from build123d import *

# Parameters (mm, degrees)
SKETCH1_R               = 2.485
SKETCH1_R_2             = 2.6
BOSS_EXTRUDE1_DEPTH     = 6
SKETCH2_R               = 2.485
BOSS_EXTRUDE2_DEPTH     = 2
SKETCH3_R               = 1.6
CUT_EXTRUDE1_DEPTH      = 10
SKETCH4_R               = 3
CUT_EXTRUDE2_DEPTH      = 28.03
BOSS_EXTRUDE3_DEPTH     = 20.015
SKETCH6_R               = 2.485
CUT_EXTRUDE3_DEPTH      = 10
CUT_EXTRUDE6_DEPTH      = 91.116192357
CUT_EXTRUDE6_DEPTH_BACK = 6
SKETCH10_R              = 1.485
SKETCH9_R               = 3
SKETCH9_R_2             = 1.485
SKETCH9_R_3             = 2.6
SKETCH9_R_4             = 1.6
CUT_EXTRUDE5_DEPTH      = 109.243744046
FILLET1_R               = 1.5


with BuildPart() as part:
    # Sketch1 → Boss-Extrude1 (new, symmetric)
    with BuildSketch(Plane(origin=(0, 0, 0), x_dir=(1, 0, 0), z_dir=(0, 1, 0))):
        with BuildLine():
            Line((20.015, -4.1), (20.015, -10.015))
            Line((20.015, -10.015), (-20.015, -10.015))
            Line((-20.015, -10.015), (-20.015, 10.015))
            Line((-20.015, 10.015), (20.015, 10.015))
            Line((20.015, 10.015), (20.015, 4.1))
            ThreePointArc((20.015, 4.1), (21.182179477, 1.282179477), (24, 0.115))
            Line((24, 0.115), (29.985, 0.115))
            Line((29.985, 0.115), (29.985, 14.015))
            Line((29.985, 14.015), (-29.985, 14.015))
            Line((-29.985, 14.015), (-29.985, 7.6))
            Line((-29.985, 7.6), (-37.485, 7.6))
            ThreePointArc((-37.485, 7.6), (-45.085, 0), (-37.485, -7.6))
            Line((-37.485, -7.6), (-29.985, -7.6))
            Line((-29.985, -7.6), (-29.985, -88.485))
            Line((-29.985, -88.485), (17.515, -88.485))
            Line((17.515, -88.485), (17.515, -78.515))
            Line((17.515, -78.515), (-20.015, -78.515))
            Line((-20.015, -78.515), (-20.015, -18.015))
            Line((-20.015, -18.015), (29.985, -18.015))
            Line((29.985, -18.015), (29.985, -0.115))
            Line((29.985, -0.115), (24, -0.115))
            ThreePointArc((24, -0.115), (21.182179477, -1.282179477), (20.015, -4.1))
        make_face()
        with Locations(Location((-24, -5, 0), (0, 0, 270))):
            Circle(SKETCH1_R, mode=Mode.SUBTRACT)
        with Locations(Location((-24, 5, 0), (0, 0, 270))):
            Circle(SKETCH1_R, mode=Mode.SUBTRACT)
        with Locations(Location((24, -5, 0), (0, 0, 270))):
            Circle(SKETCH1_R, mode=Mode.SUBTRACT)
        with Locations(Location((24, 5, 0), (0, 0, 270))):
            Circle(SKETCH1_R, mode=Mode.SUBTRACT)
        with Locations(Location((-37.485, 0, 0), (0, 0, 270))):
            Circle(SKETCH1_R_2, mode=Mode.SUBTRACT)
    extrude(amount=BOSS_EXTRUDE1_DEPTH, both=True)

    # Sketch2 → Boss-Extrude2 (add)
    with BuildSketch(Plane.XZ.offset(6)):
        with Locations(Location((24, -5, 0), (0, 0, 90))):
            Circle(SKETCH2_R)
        with Locations(Location((24, 5, 0), (0, 0, 90))):
            Circle(SKETCH2_R)
        with Locations(Location((-24, -5, 0), (0, 0, 90))):
            Circle(SKETCH2_R)
        with Locations(Location((-24, 5, 0), (0, 0, 90))):
            Circle(SKETCH2_R)
    extrude(amount=-BOSS_EXTRUDE2_DEPTH)

    # Sketch3 → Cut-Extrude1 (cut)
    with BuildSketch(Plane.XY.offset(18.015)):
        with Locations((10.015, 0)):
            Circle(SKETCH3_R)
    extrude(amount=-CUT_EXTRUDE1_DEPTH, mode=Mode.SUBTRACT)

    # Sketch4 → Cut-Extrude2 (cut)
    with BuildSketch(Plane(origin=(0, 0, -14.015), x_dir=(-1, 0, 0), z_dir=(0, 0, -1))):
        with Locations(Location((-10.015, 0, 0), (0, 0, 180))):
            Circle(SKETCH4_R)
    extrude(amount=-CUT_EXTRUDE2_DEPTH, mode=Mode.SUBTRACT)

    # Sketch5 → Boss-Extrude3 (add)
    with BuildSketch(Plane(origin=(0, 0, 0), x_dir=(0, 0, -1), z_dir=(1, 0, 0))):
        Polygon((-18.015, -6), (-10.015, -6), (-10.015, -21.5), (6.985, -21.5), (6.985, -33.5), (-18.015, -33.5), align=None)
    extrude(amount=BOSS_EXTRUDE3_DEPTH)

    # Sketch6 → Cut-Extrude3 (cut)
    with BuildSketch(Plane.XZ.offset(33.5)):
        with Locations(Location((10.015, 0, 0), (0, 0, 270))):
            Circle(SKETCH6_R)
    extrude(amount=-CUT_EXTRUDE3_DEPTH, mode=Mode.SUBTRACT)

    # Sketch10 → Cut-Extrude6 (cut, two sides: drawn at the far end of the back side and taken through both)
    with BuildSketch(Plane.XY.offset(18.015).offset(-CUT_EXTRUDE6_DEPTH_BACK)):
        with Locations((-14.485, 0)):
            Circle(SKETCH10_R)
    extrude(amount=CUT_EXTRUDE6_DEPTH + CUT_EXTRUDE6_DEPTH_BACK, mode=Mode.SUBTRACT)

    # Sketch9 → Cut-Extrude5 (cut, through all)
    # profile 1 of 3: a face of its own
    with BuildSketch(Plane(origin=(0, 0, 78.515), x_dir=(-1, 0, 0), z_dir=(0, 0, -1))):
        with Locations((14.485, 0)):
            Circle(SKETCH9_R)
        with Locations(Location((14.485, 0, 0), (0, 0, 180))):
            Circle(SKETCH9_R_2, mode=Mode.SUBTRACT)
    # profile 2 of 3: a face of its own
    with BuildSketch(Plane(origin=(0, 0, 78.515), x_dir=(-1, 0, 0), z_dir=(0, 0, -1))):
        with Locations((-10.015, 0)):
            Circle(SKETCH9_R_3)
        with Locations(Location((-10.015, 0, 0), (0, 0, 180))):
            Circle(SKETCH9_R_4, mode=Mode.SUBTRACT)
    # profile 3 of 3: a face of its own
    with BuildSketch(Plane(origin=(0, 0, 78.515), x_dir=(-1, 0, 0), z_dir=(0, 0, -1))):
        with Locations(Location((-10.015, 0, 0), (0, 0, 180))):
            Circle(SKETCH9_R_4)
    extrude(amount=-CUT_EXTRUDE5_DEPTH, mode=Mode.SUBTRACT)

    # Fillet1
    fillet1_edges = [part.edges().sort_by_distance(p)[0] for p in [
        (20.015, -6, 14.015),
        (0, -6, 14.015),
        (20.015, -27.5, -6.985),
        (0, -27.5, -6.985),
        (10.0075, -33.5, 18.015),
        (-29.985, 0, -14.015),
        (29.985, 0, -14.015),
        (29.985, 0, 18.015),
        (-20.015, 0, 18.015),
        (-20.015, 0, 78.515),
        (-29.985, 0, 88.485),
    ]]
    fillet(fillet1_edges, radius=FILLET1_R)


solid = part.part
The model under review builds one solid part; all positions refer to its coordinate system, in mm. A direction names the side the tool comes from. Round coordinates to 2 decimals unless told otherwise and drop trailing zeros. Write each loop counter-clockwise with the first axis right and the second up, starting at its lowest first coordinate (ties: lowest second). Pieces come first, ordered by that corner, then holes. Notation, with made-up numbers: (-6, 60) -> (19, 60) arc R5 ccw to (19, 68) -> close; hole circle Ø8 at (-10, 12.5). An arc over 180 degrees is marked (long way). Answer as a JSON object with one key per item and string values.
1. We need section A-A on y = -29. State the section outline as (x, z) points (3 decimals).
Results found:
{"outline": "(0, -5.485) arc R1.5 ccw to (1.5, -6.985) -> (18.515, -6.985) arc R1.5 ccw to (20.015, -5.485) -> (20.015, 18.015) -> (0, 18.015) -> close; hole circle Ø4.97 at (10.015, 0)"}
2. We need section B-B on y = 0. State how many separate pieces and enclosed holes the cut face has, and give its area (3 significant figures).
Results found:
{"separate pieces": "5", "enclosed holes": "5", "area": "2,100 mm^2"}
3. Machinability: for faces 1 (the face through (-11.488, 0.132, 83.43)), 2 (the face through (27, 0, -0.115)), 3 (the face through (25.68, 0.93, 3.17)), which of the approach directions +Z, -Z, +X, -X, +Y, -Y give a long, thin tool a straight path to every point of the face, cutting with its end or side? Answer none if there is none.
Results found:
{"face 1": "+Z", "face 2": "+X, +Y, -Y", "face 3": "+Y"}
4. Clearance check with flat-ended pins moving along their axes: pin 1 (2 mm diameter, centred on x = 16.5, y = -13, fed in from +Z) (3 decimals); pin 2 (11 mm diameter, centred on y = 2.5, z = 85.5, fed in from +X) (3 decimals); pin 3 (6.5 mm diameter, centred on x = 24, z = 5, fed in from -Y). State where each tip first meets the part, or that it passes through.
Results found:
{"pin 1": "stops at z = 18.015", "pin 2": "stops at x = 17.515", "pin 3": "stops at y = -6"}
5. We need section C-C on x = -24. State the section outline as (y, z) points (3 decimals), and give its area (3 significant figures).
Results found:
{"outline": "(-6, -14.015) -> (6, -14.015) -> (6, -7.485) -> (-4, -7.485) -> (-4, -2.515) -> (6, -2.515) -> (6, 2.515) -> (-4, 2.515) -> (-4, 7.485) -> (6, 7.485) -> (6, 88.485) -> (-6, 88.485) -> close", "area": "1,130 mm^2"}
6. The part is to be moulded in two halves that separate along Z. For faces 4 (the face through (12.612, 0.114, 83.43)), 5 (the face through (5, -9, 18.015)), 6 (the face through (10, -27, -6.985)), say which applies: pulls with the +Z half, pulls with the -Z half, needs draft (parallel to the pull), parting line crosses it, or undercut.
Results found:
{"face 4": "needs draft", "face 5": "undercut", "face 6": "pulls with the -Z half"}
7. To check wall thickness, follow line 1 along Z through (x, y) = (24, 2) (3 decimals); line 2 along X through (y, z) = (2, -5) (3 decimals); line 3 along Y through (x, z) = (17, 80.5). State the ranges of each line that lie inside material, in increasing order.
Results found:
{"line 1": "z = -14.015 to -7.485, -2.515 to -0.115, 0.115 to 2.515, 7.485 to 18.015", "line 2": "x = -43.209 to -26.485, -21.515 to -20.015, 20.015 to 21.515, 26.485 to 29.985", "line 3": "y = -6 to 6"}
8. We need section D-D on z = 72. State the section outline as (x, y) points (3 decimals).
Results found:
{"outline": "(-29.985, -6) -> (-20.015, -6) -> (-20.015, 6) -> (-29.985, 6) -> close"}
